```python
from build123d import *

# Parameters (mm, degrees)
SKETCH_1_W      = 8
SKETCH_1_H      = 8
HEIGHT_DEPTH    = 3.2
SKETCH_2_R      = 2.4
EXTRUDE_2_DEPTH = 1.7
SHELL_1_T       = -1.6


with BuildPart() as part:
    # 草圖1 → height (new body)
    with BuildSketch(Plane(origin=(0, 0, 0), x_dir=(1, 0, 0), z_dir=(0, 1, 0))):
        Rectangle(SKETCH_1_W, SKETCH_1_H)
    extrude(amount=HEIGHT_DEPTH)

    # 草圖2 → 填料-伸長2 (add)
    with BuildSketch(Plane(origin=(0, 3.2, 0), x_dir=(1, 0, 0), z_dir=(0, 1, 0))):
        Circle(SKETCH_2_R)
    extrude(amount=EXTRUDE_2_DEPTH)

    # 薄殼1
    shell_1_openings = [part.faces().sort_by_distance(p)[0] for p in [
        (0, 0, 0),
    ]]
    offset(amount=SHELL_1_T, openings=shell_1_openings, kind=Kind.INTERSECTION)


solid = part.part
```
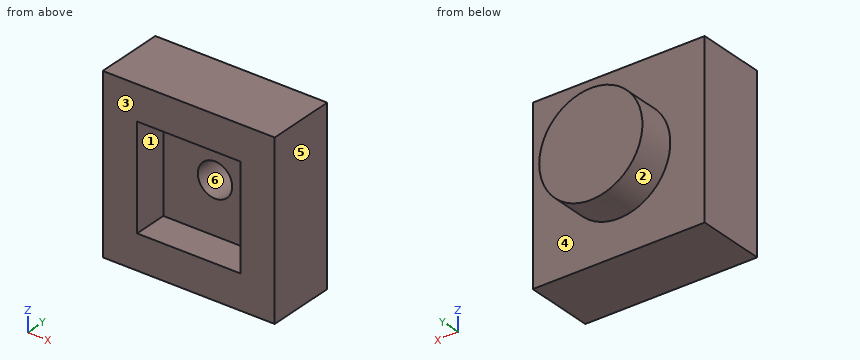
Source: CAD feature listing. Evaluate the final solid. Frame: model axes, mm. Face numbers are marked on the shaded views. A direction names the side the tool comes from. Coordinates: 2 decimals unless noted, no trailing zeros. Write each loop counter-clockwise with the first axis right and the second up, starting at its lowest first coordinate (ties: lowest second). Pieces come first, ordered by that corner, then holes. Notation, with made-up numbers: M -25,27 L 26,27 A25 ccw 26,59 Z; hole C -14.75,-9.75 d11. An arc over 180 degrees is marked long. Answer as a JSON object with one key per item and string values.
1. Access query for the marked faces 4, 5 and 6. Directions: +Z, -Z, +X, -X, +Y, -Y. A direction counts if a zero-diameter tool reaches every point of the face in a straight line with its end or side. Return the directions, or none.
Evaluation:
{"face 4": "+Y", "face 5": "+Z, -Z, +X, +Y, -Y", "face 6": "-Y"}
2. Contact query for flat-ended pins moving along their axis: P1, Ø1.4, axis at x = 0, z = 1, coming from the -Y side; P2, Ø1, axis at x = 0, z = 0, coming from the -Y side; P3, Ø3, axis at x = 2.5, z = -3, coming from the -Y side. Output: stop coordinate, or through.
Evaluation:
{"P1": "y = 1.6", "P2": "y = 3.3", "P3": "y = 0"}
3. Cut plane D-D on y = 3.75. Output: boundary loops of the cut face in (x, z), plus the area to 3 significant figures.
Evaluation:
{"outline": "C 0,0 d4.8", "area": "18.1 mm^2"}
4. Cut plane C-C on x = 0. Output: boundary loops of the cut face in (y, z), plus the area to 3 significant figures.
Evaluation:
{"outline": "M 0,-4 L 3.2,-4 L 3.2,-2.4 L 4.9,-2.4 L 4.9,2.4 L 3.2,2.4 L 3.2,4 L 0,4 L 0,2.4 L 1.6,2.4 L 1.6,0.8 L 3.3,0.8 L 3.3,-0.8 L 1.6,-0.8 L 1.6,-2.4 L 0,-2.4 Z", "area": "23.4 mm^2"}
5. Ray query, L1, parallel to Z at x = -0.25, y = 1.45; L2, parallel to Z at x = 0, y = 2.65. Return the intervals inside material, ascending.
Evaluation:
{"L1": "-4 to -2.4, 2.4 to 4", "L2": "-4 to -0.8, 0.8 to 4"}
6. Cut plane B-B on z = 0. Output: boundary loops of the cut face in (x, y).
Evaluation:
{"outline": "M -4,0 L -2.4,0 L -2.4,1.6 L -0.8,1.6 L -0.8,3.3 L 0.8,3.3 L 0.8,1.6 L 2.4,1.6 L 2.4,0 L 4,0 L 4,3.2 L 2.4,3.2 L 2.4,4.9 L -2.4,4.9 L -2.4,3.2 L -4,3.2 Z"}
7. Cut plane A-A on y = 1.5. Output: boundary loops of the cut face in (x, z), plus the area to 3 significant figures.
Evaluation:
{"outline": "M -4,-4 L 4,-4 L 4,4 L -4,4 Z; hole M -2.4,-2.4 L 2.4,-2.4 L 2.4,2.4 L -2.4,2.4 Z", "area": "41.0 mm^2"}
8. Draft query along Z for the marked faces 1, 2 and 3. Return one class per face: released by +Z, released by -Z, zero draft, split by the parting line, or undercut.
Evaluation:
{"face 1": "undercut", "face 2": "split by the parting line", "face 3": "zero draft"}
